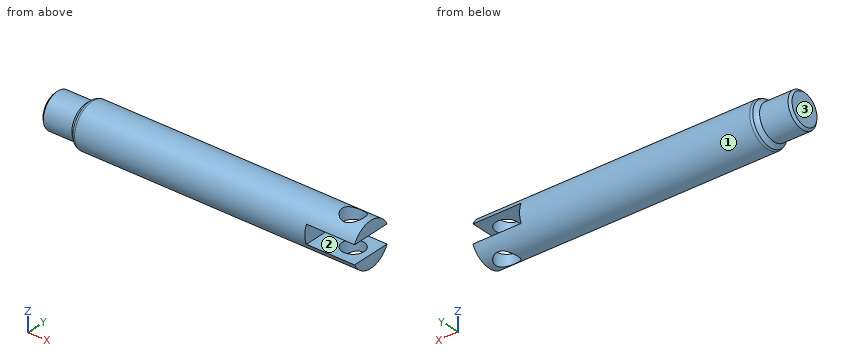
```python
from build123d import *

# Parameters (mm, degrees)
SKETCH2_W               = 2.1
SKETCH2_H               = 5.824035358
CUT_EXTRUDE1_DEPTH      = 5.5
CUT_EXTRUDE2_DEPTH      = 19.516276624
CUT_EXTRUDE2_DEPTH_BACK = 19.516276624
SKETCH3_R               = 1.25
CHAMFER1_SIZE           = 0.25
CHAMFER2_SIZE           = 0.218100459


with BuildPart() as part:
    # Sketch1 → Revolve1 (revolve)
    with BuildSketch(Plane.XY, mode=Mode.PRIVATE) as revolve1_sk:
        with BuildLine():
            Line((-18, 2), (-14.5, 2))
            ThreePointArc((-14.5, 2), (-14.208348655, 2.208348655), (-14, 2.5))
            Line((-14, 2.5), (18, 2.5))
            Line((18, 2.5), (18, 0))
            Line((18, 0), (-18, 0))
            Line((-18, 0), (-18, 2))
        make_face()
    revolve(revolve1_sk.sketch.rotate(Axis((18, 0, 0), (-1, 0, 0)), 90), axis=Axis((18, 0, 0), (-1, 0, 0)))

    # Sketch2 → Cut-Extrude1 (cut)
    with BuildSketch(Plane(origin=(18, 0, 0), x_dir=(0, 0, -1), z_dir=(1, 0, 0))):
        Rectangle(SKETCH2_W, SKETCH2_H)
    extrude(amount=-CUT_EXTRUDE1_DEPTH, mode=Mode.SUBTRACT)

    # Sketch3 → Cut-Extrude2 (cut, two sides: drawn at the far end of the back side and taken through both)
    with BuildSketch(Plane.XY.offset(-1.05).offset(-CUT_EXTRUDE2_DEPTH_BACK)):
        with Locations((15.991222224, 0)):
            Circle(SKETCH3_R)
    extrude(amount=CUT_EXTRUDE2_DEPTH + CUT_EXTRUDE2_DEPTH_BACK, mode=Mode.SUBTRACT)

    # Chamfer1
    chamfer1_edges = [part.edges().sort_by_distance(p)[0] for p in [
        (-18, 0, 2),
    ]]
    chamfer(chamfer1_edges, length=CHAMFER1_SIZE)

    # Chamfer2
    # the kernel refuses this chamfer: 0.218100459, 0.1 mm, written as the material it takes off along each edge
    with BuildSketch(Plane(origin=(-14, 0, 0), x_dir=(0, 0, -1), z_dir=(0, 1, 0))) as chamfer2_piece_1:
        with BuildLine():
            Line((2.407857149, 0.050754033), (2.5, -CHAMFER2_SIZE * 0.99999999787))
            Line((2.5, -CHAMFER2_SIZE * 0.99999999787), (2.5, 0))
            ThreePointArc((2.5, 0), (2.450478775, 0.025833705), (2.407857149, 0.050754033))
        make_face()
    revolve(axis=Axis((-14, 0, 0), (-1, 0, 0)), mode=Mode.SUBTRACT)


solid = part.part
```
Can you work these out from the model? Positions are in its coordinate system, mm. Face numbers are marked on the shaded views. Coordinates: 2 decimals unless noted, no trailing zeros. Order: outer loops, then holes, each group sorted by start corner. A loop starts at its lowest first (then second) coordinate and runs counter-clockwise, first axis right, second up.
1. I'm going to push flat-ended pins straight in: pin 1 (2 mm diameter, centred on y = 1, z = 0, fed in from +X); pin 2 (2.5 mm diameter, centred on x = 16, y = -0.5, fed in from +Z); pin 3 (2 mm diameter, centred on x = 0.5, y = -2, fed in from -Z). Where does each tip first touch, or does it pass through?
2. Thinking about a two-plate mould opening in Z: for the marked faces 1, 2 and 3, which applies, +Z half, -Z half, draft (parallel to the pull), parting line (faces both ways), or undercut?
3. If we section it at B-B (y = 0): Please give me the cut outline in (x, z), then the cut area to 3 significant figures.
4. I need wall thicknesses on line 1 (X direction, y = 0, z = -1.6); line 2 (Z direction, x = 9, y = 0.1); line 3 (Z direction, x = -4, y = -0.7). Which ranges of each line are inside material? Lowest first, please.
5. If we section it at C-C (x = -0.5): Please give me the cut outline in (y, z), then the cut area to 3 significant figures.
6. If we section it at A-A (z = 0): Please give me the cut outline in (x, y), then the cut area to 3 significant figures.
Entries:
1. pin 1: stops at x = 12.5
1. pin 2: stops at z = 2.49
1. pin 3: stops at z = -2.29
2. face 1: parting line
2. face 2: undercut
2. face 3: draft
3. outline: (-18, -1.75) - (-17.75, -2) - (-14.5, -2) arc R1.09 cw to (-14.05, -2.41) - (-13.78, -2.5) - (14.74, -2.5) - (14.74, -1.05) - (12.5, -1.05) - (12.5, 1.05) - (14.74, 1.05) - (14.74, 2.5) - (-13.78, 2.5) - (-14.05, 2.41) arc R1.09 cw to (-14.5, 2) - (-17.75, 2) - (-18, 1.75) - close; (17.24, -2.5) - (18, -2.5) - (18, -1.05) - (17.24, -1.05) - close; (17.24, 1.05) - (18, 1.05) - (18, 2.5) - (17.24, 2.5) - close
3. area: 157 mm2
4. line 1: x = -18 to 14.74, 17.24 to 18
4. line 2: z = -2.5 to 2.5
4. line 3: z = -2.4 to 2.4
5. outline: circle Ø5 at (0, 0)
5. area: 19.6 mm2
6. outline: (-18, -1.75) - (-17.75, -2) - (-14.5, -2) arc R1.09 cw to (-14.05, -2.41) - (-13.78, -2.5) - (12.5, -2.5) - (12.5, 2.5) - (-13.78, 2.5) - (-14.05, 2.41) arc R1.09 cw to (-14.5, 2) - (-17.75, 2) - (-18, 1.75) - close
6. area: 149 mm2
